Answer from the drawing. Dimensions are ordinates in mm from the lowest x, y and z of the part. A direction names the side the tool comes from. Coordinates: 2 decimals unless noted, no trailing zeros. Order: outer loops, then holes, each group sorted by start corner. A loop starts at its lowest first (then second) coordinate and runs counter-clockwise, first axis right, second up. Notation, with made-up numbers: M 1,29.25 L 41,29.25 A18 cw 41,61.25 Z; hole C 33,13.5 d9. An arc over 180 degrees is marked long. Write each question's results on one line, items separated by ' | '.
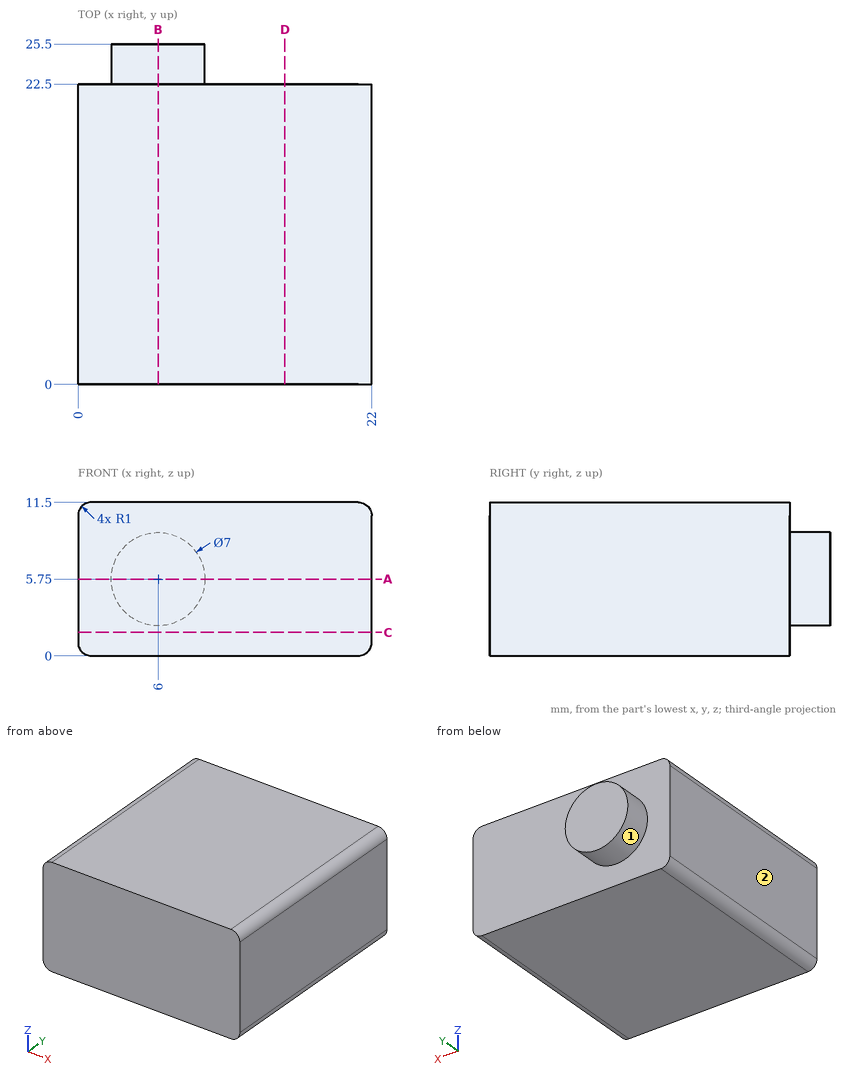
(1) The part is cut by section D-D, the plane x = 15.5. Write down the section's boundary in (y, z).
Conclusion:
outline: M 0,0 L 22.5,0 L 22.5,11.5 L 0,11.5 Z
(2) The part is cut by section B-B, the plane x = 6. Write down the section's boundary in (y, z).
Conclusion:
outline: M 0,0 L 22.5,0 L 22.5,2.25 L 25.5,2.25 L 25.5,9.25 L 22.5,9.25 L 22.5,11.5 L 0,11.5 Z
(3) Given pin 1 (12 mm diameter, centred on x = 17, y = 11, fed in from -Z); pin 2 (3.5 mm diameter, centred on x = 15.5, z = 6.5, fed in from +Y), each flat-ended and moving along its own axis, determine where each tip first touches the part or whether it passes through.
Conclusion:
pin 1: z = 0 | pin 2: y = 22.5
(4) The part is cut by section A-A, the plane z = 5.75. Write down the section's boundary in (x, y), then the cut area to 3 significant figures.
Conclusion:
outline: M 0,0 L 22,0 L 22,22.5 L 9.5,22.5 L 9.5,25.5 L 2.5,25.5 L 2.5,22.5 L 0,22.5 Z | area: 516 mm²
(5) For the marked faces 1 and 2, determine the directions among +Z, -Z, +X, -X, +Y, -Y from which every point of the face is accessible in a straight line to the end or side of a thin tool.
Conclusion:
face 1: +Y | face 2: +Z, -Z, -X, +Y, -Y
(6) Straight lines are drawn through the part: line 1 (Y direction, x = 12.5, z = 9); line 2 (X direction, y = 13.25, z = 0.75); line 3 (Z direction, x = 4.25, y = 23.25). For each, find the intervals that lie inside material, in ascending order.
Conclusion:
line 1: 0 to 22.5 | line 2: 0.03 to 21.97 | line 3: 2.72 to 8.78
(7) The part is cut by section C-C, the plane z = 1.75. Write down the section's boundary in (x, y), then the cut area to 3 significant figures.
Conclusion:
outline: M 0,0 L 22,0 L 22,22.5 L 0,22.5 Z | area: 495 mm²
